The drawing under review shows one solid part. Ordinate dimensions are in mm from its lowest x, y, z. Give positions to 0.01 mm unless a question says otherwise; leave off trailing zeros. Order: outer loops, then holes, each group sorted by start corner. A loop starts at its lowest first (then second) coordinate and runs counter-clockwise, first axis right, second up. Notation, with made-up numbers: (-25, 77) -> (2, 77) arc R18 ccw to (2, 90) -> close; hole circle Ø9 at (46.25, 68.25). An arc over 180 degrees is marked (long way). Use a Markdown table: item, result. Add a question column.
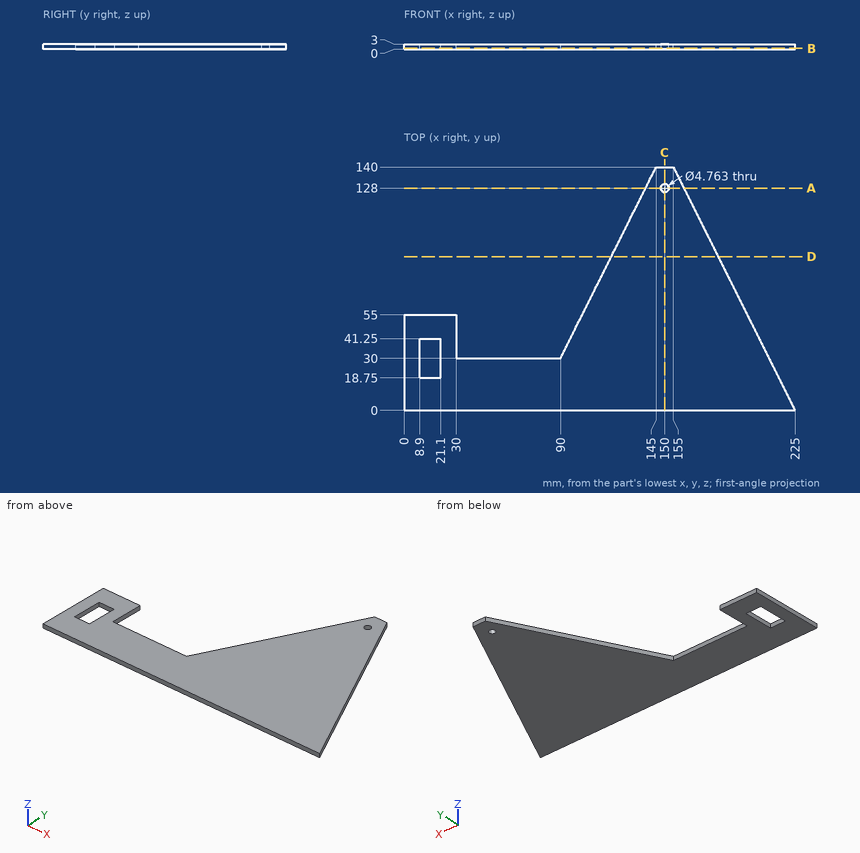
1) Add section B-B (z = 0.45). Give the boundary of the cut face in (x, y).
2) Add section C-C (x = 150). Give the boundary of the cut face in (y, z).
3) Add section A-A (y = 128). Give the boundary of the cut face in (x, z).
4) Insertion check: pin 1 (1.5 mm diameter, centred on y = 90, z = 2.5, fed in from +X) (1 decimal); pin 2 (1.5 mm diameter, centred on x = 8.5, z = 2, fed in from +Y); pin 3 (0.9 mm diameter, centred on y = 37, z = 2, fed in from +X) (1 decimal). Each pin has a flat end and moves straight along its axis. Give the tip position at first contact, or say it passes through.
5) Add section D-D (y = 88.5). Give the boundary of the cut face in (x, z).
6) For L1, parallel to Y at x = 150, z = 0.8; L2, parallel to X at y = 21, z = 0.3; L3, parallel to Y at x = 54, z = 0.55, list the stretches that pass through material, from the lowest coordinate up. Write a range as [from, to].
Worked answers:
| question | item | result |
|---|---|---|
| 1 | outline | (0, 0) -> (225, 0) -> (155, 140) -> (145, 140) -> (90, 30) -> (30, 30) -> (30, 55) -> (0, 55) -> close; hole (8.9, 18.75) -> (21.1, 18.75) -> (21.1, 41.25) -> (8.9, 41.25) -> close; hole circle Ø4.76 at (150, 128) |
| 2 | outline | (0, 0) -> (125.62, 0) -> (125.62, 3) -> (0, 3) -> close; (130.38, 0) -> (140, 0) -> (140, 3) -> (130.38, 3) -> close |
| 3 | outline | (139, 0) -> (147.62, 0) -> (147.62, 3) -> (139, 3) -> close; (152.38, 0) -> (161, 0) -> (161, 3) -> (152.38, 3) -> close |
| 4 | pin 1 | x = 180.4 |
| 4 | pin 2 | y = 55 |
| 4 | pin 3 | x = 206.7 |
| 5 | outline | (119.25, 0) -> (180.75, 0) -> (180.75, 3) -> (119.25, 3) -> close |
| 6 | L1 | [0, 125.62], [130.38, 140] |
| 6 | L2 | [0, 8.9], [21.1, 214.5] |
| 6 | L3 | [0, 30] |
